Input: part model. Units: mm. Frame: model coordinates. A direction names the side the tool comes from. Round coordinates to 2 decimals unless told otherwise and drop trailing zeros. Write each loop counter-clockwise with the first axis right and the second up, starting at its lowest first coordinate (ties: lowest second). Pieces come first, ordered by that corner, then holes. Notation, with made-up numbers: (-27, 61.25) - (30, 61.25) arc R11 ccw to (30, 69.25) - close; hole circle Ø9 at (64, 38). An arc over 180 degrees is marked (long way). Use one line per item in the form item = value.
```python
from build123d import *

# Parameters (mm, degrees)
F0_W     = 65
F0_H     = 35
F0_R     = 1.3
F1_DEPTH = 1.75
F2_W     = 2
F2_H     = 15
F3_DEPTH = 20.5
F4_W     = 10
F4_H     = 18
F5_DEPTH = 20.5


with BuildPart() as f1:
    # F0 (on Top) → F1 (new body)
    with BuildSketch(Plane.XY):
        Rectangle(F0_W, F0_H)
        with Locations((-30, -15)):
            Circle(F0_R, mode=Mode.SUBTRACT)
        with Locations((30, -15)):
            Circle(F0_R, mode=Mode.SUBTRACT)
        with Locations((-30, 15)):
            Circle(F0_R, mode=Mode.SUBTRACT)
        with Locations((30, 15)):
            Circle(F0_R, mode=Mode.SUBTRACT)
    extrude(amount=F1_DEPTH)

    # F2 (on face) → F3 (join)
    with BuildSketch(Plane.XY.offset(1.75)):
        with Locations((-27.1, 20.75)):
            Rectangle(F2_W, F2_H)
        Polygon((-26.1, 13.25), (-28.1, 13.25), (-28.1, 11.25), (28.1, 11.25), (28.1, 13.25), (26.1, 13.25), (19.066667, 13.25), (17.066667, 13.25), (10.033333, 13.25), (8.033333, 13.25), (1, 13.25), (-1, 13.25), (-8.033333, 13.25), (-10.033333, 13.25), (-17.066667, 13.25), (-19.066667, 13.25), align=None)
        with Locations((-18.066667, 20.75)):
            Rectangle(F2_W, F2_H)
        with Locations((27.1, 20.75)):
            Rectangle(F2_W, F2_H)
        with Locations((-9.033333, 20.75)):
            Rectangle(F2_W, F2_H)
        with Locations((18.066667, 20.75)):
            Rectangle(F2_W, F2_H)
        with Locations((0, 20.75)):
            Rectangle(F2_W, F2_H)
        with Locations((9.033333, 20.75)):
            Rectangle(F2_W, F2_H)
        with Locations((-9.033333, -20.75)):
            Rectangle(F2_W, F2_H)
        Polygon((-17.066667, -13.25), (-10.033333, -13.25), (-8.033333, -13.25), (-1, -13.25), (1, -13.25), (8.033333, -13.25), (10.033333, -13.25), (17.066667, -13.25), (19.066667, -13.25), (26.1, -13.25), (28.1, -13.25), (28.1, -11.25), (-28.1, -11.25), (-28.1, -13.25), (-26.1, -13.25), (-19.066667, -13.25), align=None)
        with Locations((-18.066667, -20.75)):
            Rectangle(F2_W, F2_H)
        with Locations((0, -20.75)):
            Rectangle(F2_W, F2_H)
        with Locations((-27.1, -20.75)):
            Rectangle(F2_W, F2_H)
        with Locations((9.033333, -20.75)):
            Rectangle(F2_W, F2_H)
        with Locations((18.066667, -20.75)):
            Rectangle(F2_W, F2_H)
        with Locations((27.1, -20.75)):
            Rectangle(F2_W, F2_H)
    extrude(amount=F3_DEPTH)

    # F4 (on face) → F5 (join, through all)
    with BuildSketch(Plane.XY.offset(1.75)):
        with Locations((32.5, 0)):
            Rectangle(F4_W, F4_H)
    extrude(amount=F5_DEPTH)


solid = f1.part
```
(1) Cut plane D-D on y = -7. Output: boundary loops of the cut face in (x, z), then the cut area to 3 significant figures.
Derived:
outline = (-32.5, 0) - (32.5, 0) - (32.5, 1.75) - (37.5, 1.75) - (37.5, 22.25) - (27.5, 22.25) - (27.5, 1.75) - (-32.5, 1.75) - close
area = 319 mm^2
(2) Material intervals for L1, parallel to Y at x = 30, z = 1.45; L2, parallel to Y at x = 19, z = 12.25; L3, parallel to Y at x = 2, z = 18.75, sorted ascending.
Derived:
L1 = -17.5 to -16.3, -13.7 to 13.7, 16.3 to 17.5
L2 = -28.25 to -11.25, 11.25 to 28.25
L3 = -13.25 to -11.25, 11.25 to 13.25
(3) Cut plane C-C on x = 7. Output: boundary loops of the cut face in (y, z), then the cut area to 3 significant figures.
Derived:
outline = (-17.5, 0) - (17.5, 0) - (17.5, 1.75) - (13.25, 1.75) - (13.25, 22.25) - (11.25, 22.25) - (11.25, 1.75) - (-11.25, 1.75) - (-11.25, 22.25) - (-13.25, 22.25) - (-13.25, 1.75) - (-17.5, 1.75) - close
area = 143 mm^2
(4) Cut plane A-A on y = 19. Output: boundary loops of the cut face in (x, z), then the cut area to 3 significant figures.
Derived:
outline = (-28.1, 1.75) - (-26.1, 1.75) - (-26.1, 22.25) - (-28.1, 22.25) - close; (-19.07, 1.75) - (-17.07, 1.75) - (-17.07, 22.25) - (-19.07, 22.25) - close; (-10.03, 1.75) - (-8.03, 1.75) - (-8.03, 22.25) - (-10.03, 22.25) - close; (-1, 1.75) - (1, 1.75) - (1, 22.25) - (-1, 22.25) - close; (8.03, 1.75) - (10.03, 1.75) - (10.03, 22.25) - (8.03, 22.25) - close; (17.07, 1.75) - (19.07, 1.75) - (19.07, 22.25) - (17.07, 22.25) - close; (26.1, 1.75) - (28.1, 1.75) - (28.1, 22.25) - (26.1, 22.25) - close
area = 287 mm^2
(5) Access query for faces 1 (the face through (-18, -28.25, 12)), 2 (the face through (-5, 15, 1.75)), 3 (the face through (14, -15, 1.75)), 4 (the face through (28.7, -14.94, 0.86)), 5 (the face through (9, -23, 1.75)). Directions: +Z, -Z, +X, -X, +Y, -Y. A direction counts if a zero-diameter tool reaches every point of the face in a straight line with its end or side. Return the directions, or none.
Derived:
face_1 = +Z, -Z, +X, -X, -Y
face_2 = +Z, +Y
face_3 = +Z, -Y
face_4 = +Z, -Z
face_5 = -Z, +X, -X, -Y
(6) Draft query along X for faces 6 (the face through (-18, -23, 1.75)), 7 (the face through (28.7, 15.06, 0.86)), 8 (the face through (28.1, -20, 12)). Return one class per face: released by +X, released by -X, zero draft, split by the parting line, or undercut.
Derived:
face_6 = zero draft
face_7 = undercut
face_8 = released by +X
(7) Cut plane B-B on x = 30. Output: boundary loops of the cut face in (y, z).
Derived:
outline = (-17.5, 0) - (-16.3, 0) - (-16.3, 1.75) - (-17.5, 1.75) - close; (-13.7, 0) - (13.7, 0) - (13.7, 1.75) - (9, 1.75) - (9, 22.25) - (-9, 22.25) - (-9, 1.75) - (-13.7, 1.75) - close; (16.3, 0) - (17.5, 0) - (17.5, 1.75) - (16.3, 1.75) - close
(8) First-contact query: pin 1 Ø4 at (y, z) = (11.5, 5) entering from -X; pin 2 Ø2 at (x, y) = (6, 15.5) entering from +Z; pin 3 Ø0.6 at (x, y) = (27, 20.5) entering from -Z. Flat tips, straight axial feed; report the tip coordinate or a pass-through.
Derived:
pin_1 = -28.1
pin_2 = 1.75
pin_3 = 1.75
